from build123d import *

# Parameters (mm, degrees)
SKETCH1_R               = 5
BOSS_EXTRUDE1_DEPTH     = 25
CUT_EXTRUDE1_DEPTH      = 35
CUT_EXTRUDE1_DEPTH_BACK = 15
SKETCH2_W               = 15
SKETCH2_H               = 290
SKETCH3_R               = 5
CUT_EXTRUDE4_DEPTH      = 40
SKETCH7_W               = 25
SKETCH7_H               = 28.664698835
CUT_EXTRUDE7_DEPTH      = 30
SKETCH9_R               = 2.5
BOSS_EXTRUDE3_DEPTH     = 5


with BuildPart() as part:
    # Sketch1 → Boss-Extrude1 (new body)
    with BuildSketch(Plane(origin=(0, 0, 0), x_dir=(0, 0, -1), z_dir=(1, 0, 0))):
        with BuildLine():
            Line((-150.552761917, 18.987019815), (149.447238083, 21.532711721))
            ThreePointArc((149.447238083, 21.532711721), (162.052854746, 9.139228412), (149.659371437, -3.466388252))
            Line((149.659371437, -3.466388252), (-150.340628563, -6.012080158))
            ThreePointArc((-150.340628563, -6.012080158), (-162.946245226, 6.381403151), (-150.552761917, 18.987019815))
        make_face()
        with Locations((149.55330476, 9.033161734)):
            Circle(SKETCH1_R, mode=Mode.SUBTRACT)
    extrude(amount=BOSS_EXTRUDE1_DEPTH)

    # Sketch2 → Cut-Extrude1 (cut, two sides: drawn at the far end of the back side and taken through both)
    with BuildSketch(Plane(origin=(0, 0, 0), x_dir=(1, 0, 0), z_dir=(0, 1, 0)).offset(-CUT_EXTRUDE1_DEPTH_BACK)):
        with Locations((12.5, 22.738394002)):
            Rectangle(SKETCH2_W, SKETCH2_H)
    extrude(amount=CUT_EXTRUDE1_DEPTH + CUT_EXTRUDE1_DEPTH_BACK, mode=Mode.SUBTRACT)

    # Sketch3 → Cut-Extrude4 (cut)
    with BuildSketch(Plane(origin=(25, 0, 0), x_dir=(0, 0, -1), z_dir=(1, 0, 0))):
        with Locations((-150.44669524, 6.487469828)):
            Circle(SKETCH3_R)
    extrude(amount=-CUT_EXTRUDE4_DEPTH, mode=Mode.SUBTRACT)

    # Sketch7 → Cut-Extrude7 (cut)
    with BuildSketch(Plane(origin=(0, -1.382144103, 162.880366562), x_dir=(1, 0, 0), z_dir=(0, -0.008485334194353043, 0.9999639989037656))):
        with Locations((12.5, 7.004905365)):
            Rectangle(SKETCH7_W, SKETCH7_H)
    extrude(amount=-CUT_EXTRUDE7_DEPTH, mode=Mode.SUBTRACT)

    # Sketch9 → Boss-Extrude3 (add)
    with BuildSketch(Plane(origin=(0, -1.127584077, 132.881446595), x_dir=(1, 0, 0), z_dir=(0, -0.008485334194353164, 0.9999639989037656))):
        with Locations(Location((12.5, 7.76382676, 0), (0, 0, 270))):
            Circle(SKETCH9_R)
    extrude(amount=BOSS_EXTRUDE3_DEPTH)


solid = part.part
Geometry: final body of the model. Coordinates: model frame, mm. A direction names the side the tool comes from. Give positions to 0.01 mm unless a question says otherwise; leave off trailing zeros. Order: outer loops, then holes, each group sorted by start corner. A loop starts at its lowest first (then second) coordinate and runs counter-clockwise, first axis right, second up. Notation, with made-up numbers: (-19.5, 45) -> (6.5, 45) arc R28 ccw to (6.5, 65) -> close; hole circle Ø1 at (61.5, 47). An arc over 180 degrees is marked (long way). Answer as a JSON object with one key per item and string values.
Q1. Draft query along X for faces 1 (the cylindrical face through (10.06, 7.16, 135.42)), 2 (the cylindrical face through (2.46, 10.54, -154.32)), 3 (the flat face through (5, 8, -18)). Return one class per face: released by +X, released by -X, zero draft, split by the parting line, or undercut.
Entries:
{"face 1": "split by the parting line", "face 2": "zero draft", "face 3": "undercut"}
Q2. Section B-B (y = 1). Output: boundary loops of the cut face in (x, z).
Entries:
{"outline": "(0, -159.13) -> (5, -159.13) -> (5, 122.26) -> (20, 122.26) -> (20, -159.13) -> (25, -159.13) -> (25, 132.9) -> (0, 132.9) -> close"}
Q3. Access query for faces 4 (the cylindrical face through (22.46, 10.54, -154.32)), 5 (the flat face through (20, 8, -18)). Directions: +Z, -Z, +X, -X, +Y, -Y. A direction counts if a zero-diameter tool reaches every point of the face in a straight line with its end or side. Return the directions, or none.
Entries:
{"face 4": "+X, -X", "face 5": "-Z, +Y, -Y"}
Q4. Material intervals for probe 1 along X at (y, z) = (-2, 15); probe 2 along Z at (x, y) = (16.75, 0.5); probe 3 along Z at (x, y) = (12.75, 14.5), sorted ascending.
Entries:
{"probe 1": "x = 0 to 5, 20 to 25", "probe 2": "z = 122.26 to 132.9", "probe 3": "z = 122.26 to 133.01"}
Q5. First-contact query: pin 1 (3 mm diameter, centred on x = 2.5, y = 2, fed in from +Z); pin 2 (12 mm diameter, centred on x = 7, y = 15.5, fed in from +Z); pin 3 (3 mm diameter, centred on x = 16, y = 6.5, fed in from +Z); pin 4 (6 mm diameter, centred on y = 9.03, z = -149.55, fed in from +X). Flat tips, straight axial feed; report the tip coordinate or a pass-through.
Entries:
{"pin 1": "stops at z = 132.92", "pin 2": "stops at z = 133.05", "pin 3": "stops at z = 137.95", "pin 4": "passes through"}
Q6. Section A-A (z = 97.5). Output: boundary loops of the cut face in (x, y).
Entries:
{"outline": "(0, -5.56) -> (5, -5.56) -> (5, 19.44) -> (0, 19.44) -> close; (20, -5.56) -> (25, -5.56) -> (25, 19.44) -> (20, 19.44) -> close"}
